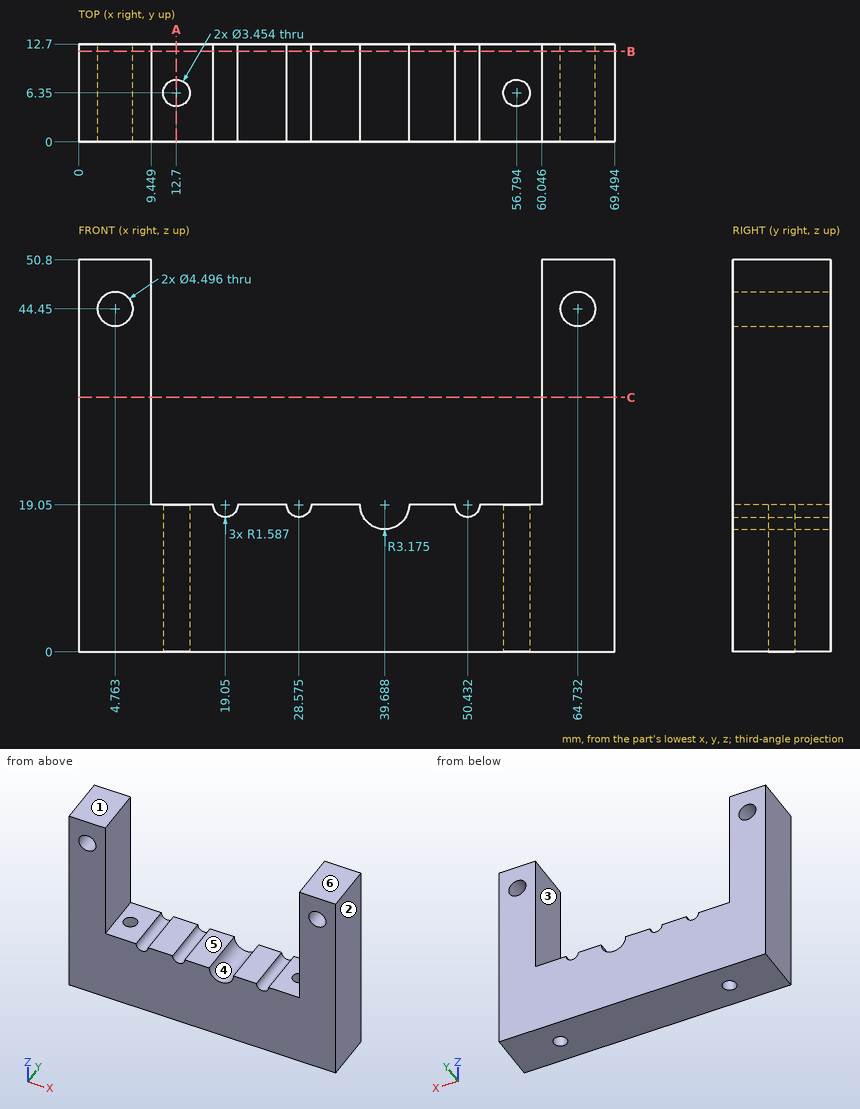
Input: dimensioned drawing with shaded views. Units: mm. Origin: part minimum x, y, z. A direction names the side the tool comes from. Coordinates: 2 decimals unless noted, no trailing zeros. Loops run counter-clockwise (first coordinate to the right, second up) from the corner with the lowest first, then second, coordinate; pieces in that order, holes last. Notation, with made-up numbers: M 42,89.5 L 70,89.5 A4 cw 70,94.5 Z; hole C -8.5,-18 d6. An arc over 180 degrees is marked long. Use a Markdown table: item, result. Add a question column.
Q1. Draft query along X for the marked faces 1, 2, 3 and 4. Return one class per face: pulls with the +X half, pulls with the -X half, needs draft (parallel to the pull), parting line crosses it, or undercut.
Q2. Section query B-B, the plane y = 11.75. State how many separate pieces and enclosed holes the cut face has, and give its area (3 significant figures).
Q3. Access query for the marked faces 5 and 6. Directions: +Z, -Z, +X, -X, +Y, -Y. A direction counts if a zero-diameter tool reaches every point of the face in a straight line with its end or side. Return the directions, or none.
Q4. Section query A-A, the plane x = 12.7. Return loops of the section in (y, z), and give its area (3 significant figures).
Q5. Section query C-C, the plane z = 33. Return loops of the section in (x, y) (1 decimal).
Q6. Material intervals for L1, parallel to X at y = 5, z = 31 (1 decimal); L2, parallel to X at y = 5.5, z = 16.5 (1 decimal); L3, parallel to Z at x = 26.5, y = 9, sorted ascending.
Q7. First-contact query: pin 1 (3 mm diameter, centred on x = 33.5, y = 4.5, fed in from +Z); pin 2 (4 mm diameter, centred on x = 64.73, z = 44.45, fed in from -Y); pin 3 (1.5 mm diameter, centred on x = 29, y = 5.5, fed in from +Z). Flat tips, straight axial feed; report the tip coordinate or a pass-through.
Result:
| question | item | result |
|---|---|---|
| 1 | face 1 | needs draft |
| 1 | face 2 | pulls with the +X half |
| 1 | face 3 | undercut |
| 1 | face 4 | undercut |
| 2 | separate pieces | 1 |
| 2 | enclosed holes | 2 |
| 2 | area | 1,860 mm2 |
| 3 | face 5 | +Z, +Y, -Y |
| 3 | face 6 | +Z, +X, -X, +Y, -Y |
| 4 | outline | M 0,0 L 4.62,0 L 4.62,19.05 L 0,19.05 Z; M 8.08,0 L 12.7,0 L 12.7,19.05 L 8.08,19.05 Z |
| 4 | area | 176 mm2 |
| 5 | outline | M 0,0 L 9.4,0 L 9.4,12.7 L 0,12.7 Z; M 60,0 L 69.5,0 L 69.5,12.7 L 60,12.7 Z |
| 6 | L1 | x = 0 to 9.4, 60 to 69.5 |
| 6 | L2 | x = 0 to 11.2, 14.2 to 37.8, 41.6 to 55.3, 58.3 to 69.5 |
| 6 | L3 | z = 0 to 19.05 |
| 7 | pin 1 | stops at z = 19.05 |
| 7 | pin 2 | passes through |
| 7 | pin 3 | stops at z = 17.98 |
